Check sheet for the modelled part. Datum: model origin and axes. Units: mm. Round coordinates to 2 decimals unless told otherwise and drop trailing zeros. Loops run counter-clockwise (first coordinate to the right, second up) from the corner with the lowest first, then second, coordinate; pieces in that order, holes last. Notation, with made-up numbers: (79, 42.5) -> (123, 42.5) arc R8 cw to (123, 57.5) -> close; hole circle Ø5 at (-17, 10). An arc over 180 degrees is marked (long way). Use one line per item in the form item = value. Start each with the question number.
(1) Sectioned sample at A-A (y = -50). Record the cut outline in (x, z), and give its area (3 significant figures).
(2) Sectioned sample at D-D (x = 0). State how many separate pieces and enclosed holes the cut face has, and give its area (3 significant figures).
(3) Go/stop test with flat-tipped pins: pin 1 (2.5 mm diameter, centred on x = 0, y = -16.5, fed in from -Z); pin 2 (3 mm diameter, centred on x = -10, z = 4.5, fed in from -Y); pin 3 (3 mm diameter, centred on x = -14, z = 2, fed in from +Y); pin 4 (6 mm diameter, centred on x = 0, y = -50, fed in from -Z). Record where each tip stops, or that it passes through.
(4) Material ranges on probe 1 along Y at (x, z) = (-30, 1.75); probe 2 along Y at (x, z) = (-50, 2.85); probe 3 along X at (y, z) = (20, 4.75), recorded low to high. Write a range as [from, to].
(5) Sectioned sample at C-C (x = -16.5). Record the cut outline in (y, z).
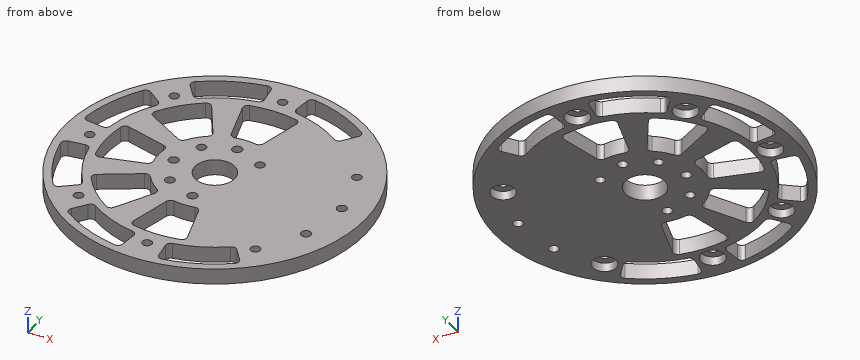
from build123d import *

# Parameters (mm, degrees)
SKETCH1_R                = 60.5
SKETCH1_R_2              = 1.89865
SKETCH1_R_3              = 1.9939
SKETCH1_R_4              = 8
BOSS_EXTRUDE1_DEPTH      = 6.35
CUT_EXTRUDE1_DEPTH       = 86.795235882
FILLET1_R                = 2
CIRPATTERN1_COUNT        = 8
FILLET1_OF_CIRPATTERN1_R = 2
CUT_EXTRUDE2_DEPTH       = 86.795235882
FILLET2_R                = 2
CIRPATTERN3_COUNT        = 8
FILLET2_OF_CIRPATTERN3_R = 2
SKETCH4_R                = 4.7625
SKETCH4_R_2              = 1.89865
CUT_EXTRUDE3_DEPTH       = 3.571875


with BuildPart() as part:
    # Sketch1 → Boss-Extrude1 (new body)
    with BuildSketch(Plane.XY):
        Circle(SKETCH1_R)
        with Locations((45.315389352, 21.130913087)):
            Circle(SKETCH1_R_2, mode=Mode.SUBTRACT)
        with Locations((49.978847504, 1.454235937)):
            Circle(SKETCH1_R_3, mode=Mode.SUBTRACT)
        Circle(SKETCH1_R_4, mode=Mode.SUBTRACT)
        with Locations((46.467376211, -18.460307366)):
            Circle(SKETCH1_R_3, mode=Mode.SUBTRACT)
        with Locations((0, -16.5)):
            Circle(SKETCH1_R_3, mode=Mode.SUBTRACT)
        with Locations((0, -50)):
            Circle(SKETCH1_R_2, mode=Mode.SUBTRACT)
        with Locations((-16.5, 0)):
            Circle(SKETCH1_R_3, mode=Mode.SUBTRACT)
        with Locations((-11.66726189, -11.66726189)):
            Circle(SKETCH1_R_2, mode=Mode.SUBTRACT)
        with Locations((0, 16.5)):
            Circle(SKETCH1_R_3, mode=Mode.SUBTRACT)
        with Locations((-11.66726189, 11.66726189)):
            Circle(SKETCH1_R_2, mode=Mode.SUBTRACT)
        with Locations((11.66726189, 11.66726189)):
            Circle(SKETCH1_R_2, mode=Mode.SUBTRACT)
        with Locations((-35.355339059, -35.355339059)):
            Circle(SKETCH1_R_2, mode=Mode.SUBTRACT)
        with Locations((-50, 0)):
            Circle(SKETCH1_R_2, mode=Mode.SUBTRACT)
        with Locations((-35.355339059, 35.355339059)):
            Circle(SKETCH1_R_2, mode=Mode.SUBTRACT)
        with Locations((0, 50)):
            Circle(SKETCH1_R_2, mode=Mode.SUBTRACT)
        with Locations((35.355339059, -35.355339059)):
            Circle(SKETCH1_R_2, mode=Mode.SUBTRACT)
    extrude(amount=BOSS_EXTRUDE1_DEPTH)

    # Sketch2 → Cut-Extrude1 (cut, through all)
    with BuildSketch(Plane.XY.offset(6.35)):
        with BuildLine():
            Line((-22.071405131, 5.914015181), (-42.162662318, 11.297451319))
            ThreePointArc((-42.162662318, 11.297451319), (-43.65, 0), (-42.162662318, -11.297451319))
            Line((-42.162662318, -11.297451319), (-22.071405131, -5.914015181))
            ThreePointArc((-22.071405131, -5.914015181), (-22.85, 0), (-22.071405131, 5.914015181))
        make_face()
    cut_extrude1 = extrude(amount=-CUT_EXTRUDE1_DEPTH, mode=Mode.SUBTRACT)

    # Fillet1
    fillet1_edges = [part.edges().sort_by_distance(p)[0] for p in [
        (-42.162662318, -11.297451319, 3.175),
        (-42.162662318, 11.297451319, 3.175),
        (-22.071405131, 5.914015181, 3.175),
        (-22.071405131, -5.914015181, 3.175),
    ]]
    fillet(fillet1_edges, radius=FILLET1_R)

    # CirPattern1: Cut-Extrude1 ×8 about axis, 3 skipped
    cirpattern1_axis = Axis((0, 0, 0), (0, 0, -1))
    add([cut_extrude1.rotate(cirpattern1_axis, i * 360 / CIRPATTERN1_COUNT) for i in range(1, CIRPATTERN1_COUNT) if i not in (3, 4, 5)], mode=Mode.SUBTRACT)

    # Fillet1 of CirPattern1
    fillet1_of_cirpattern1_edges = [part.edges().sort_by_distance(p)[0] for p in [
        (-37.802008875, 21.825, 3.175),
        (-21.825, 37.802008875, 3.175),
        (-11.425, 19.788680476, 3.175),
        (-19.788680476, 11.425, 3.175),
        (-11.297451319, 42.162662318, 3.175),
        (11.297451319, 42.162662318, 3.175),
        (5.914015181, 22.071405131, 3.175),
        (-5.914015181, 22.071405131, 3.175),
        (11.297451319, -42.162662318, 3.175),
        (-11.297451319, -42.162662318, 3.175),
        (-5.914015181, -22.071405131, 3.175),
        (5.914015181, -22.071405131, 3.175),
        (-21.825, -37.802008875, 3.175),
        (-37.802008875, -21.825, 3.175),
        (-19.788680476, -11.425, 3.175),
        (-11.425, -19.788680476, 3.175),
    ]]
    fillet(fillet1_of_cirpattern1_edges, radius=FILLET1_OF_CIRPATTERN1_R)

    # Sketch3 → Cut-Extrude2 (cut, through all)
    with BuildSketch(Plane.XY.offset(6.35)):
        with BuildLine():
            Line((-45.478980232, 34.897248918), (-37.148770159, 28.505253913))
            ThreePointArc((-37.148770159, 28.505253913), (-43.26065911, 17.91915172), (-46.424405634, 6.111888951))
            Line((-46.424405634, 6.111888951), (-56.834576678, 7.482413969))
            ThreePointArc((-56.834576678, 7.482413969), (-52.961394201, 21.93732776), (-45.478980232, 34.897248918))
        make_face()
    cut_extrude2 = extrude(amount=-CUT_EXTRUDE2_DEPTH, mode=Mode.SUBTRACT)

    # Fillet2
    fillet2_edges = [part.edges().sort_by_distance(p)[0] for p in [
        (-56.834576678, 7.482413969, 3.175),
        (-45.478980232, 34.897248918, 3.175),
        (-37.148770159, 28.505253913, 3.175),
        (-46.424405634, 6.111888951, 3.175),
    ]]
    fillet(fillet2_edges, radius=FILLET2_R)

    # CirPattern3: Cut-Extrude2 ×8 about axis, 2 skipped
    cirpattern3_axis = Axis((0, 0, 0), (0, 0, -1))
    add([cut_extrude2.rotate(cirpattern3_axis, i * 360 / CIRPATTERN3_COUNT) for i in range(1, CIRPATTERN3_COUNT) if i not in (3, 4)], mode=Mode.SUBTRACT)

    # Fillet2 of CirPattern3
    fillet2_of_cirpattern3_edges = [part.edges().sort_by_distance(p)[0] for p in [
        (-34.897248918, 45.478980232, 3.175),
        (-7.482413969, 56.834576678, 3.175),
        (-6.111888951, 46.424405634, 3.175),
        (-28.505253913, 37.148770159, 3.175),
        (7.482413969, 56.834576678, 3.175),
        (34.897248918, 45.478980232, 3.175),
        (28.505253913, 37.148770159, 3.175),
        (6.111888951, 46.424405634, 3.175),
        (34.897248918, -45.478980232, 3.175),
        (7.482413969, -56.834576678, 3.175),
        (6.111888951, -46.424405634, 3.175),
        (28.505253913, -37.148770159, 3.175),
        (-7.482413969, -56.834576678, 3.175),
        (-34.897248918, -45.478980232, 3.175),
        (-28.505253913, -37.148770159, 3.175),
        (-6.111888951, -46.424405634, 3.175),
        (-45.478980232, -34.897248918, 3.175),
        (-56.834576678, -7.482413969, 3.175),
        (-46.424405634, -6.111888951, 3.175),
        (-37.148770159, -28.505253913, 3.175),
    ]]
    fillet(fillet2_of_cirpattern3_edges, radius=FILLET2_OF_CIRPATTERN3_R)

    # Sketch4 → Cut-Extrude3 (cut)
    # profile 1 of 7: a face of its own
    with BuildSketch(Plane(origin=(0, 0, 0), x_dir=(-1, 0, 0), z_dir=(0, 0, -1))):
        with Locations((0, 50)):
            Circle(SKETCH4_R)
        with Locations((0, 50)):
            Circle(SKETCH4_R_2, mode=Mode.SUBTRACT)
    # profile 2 of 7: a face of its own
    with BuildSketch(Plane(origin=(0, 0, 0), x_dir=(-1, 0, 0), z_dir=(0, 0, -1))):
        with Locations((35.355339059, 35.355339059)):
            Circle(SKETCH4_R)
        with Locations((35.355339059, 35.355339059)):
            Circle(SKETCH4_R_2, mode=Mode.SUBTRACT)
    # profile 3 of 7: a face of its own
    with BuildSketch(Plane(origin=(0, 0, 0), x_dir=(-1, 0, 0), z_dir=(0, 0, -1))):
        with Locations((50, 0)):
            Circle(SKETCH4_R)
        with Locations((50, 0)):
            Circle(SKETCH4_R_2, mode=Mode.SUBTRACT)
    # profile 4 of 7: a face of its own
    with BuildSketch(Plane(origin=(0, 0, 0), x_dir=(-1, 0, 0), z_dir=(0, 0, -1))):
        with Locations((35.355339059, -35.355339059)):
            Circle(SKETCH4_R)
        with Locations((35.355339059, -35.355339059)):
            Circle(SKETCH4_R_2, mode=Mode.SUBTRACT)
    # profile 5 of 7: a face of its own
    with BuildSketch(Plane(origin=(0, 0, 0), x_dir=(-1, 0, 0), z_dir=(0, 0, -1))):
        with Locations((0, -50)):
            Circle(SKETCH4_R)
        with Locations((0, -50)):
            Circle(SKETCH4_R_2, mode=Mode.SUBTRACT)
    # profile 6 of 7: a face of its own
    with BuildSketch(Plane(origin=(0, 0, 0), x_dir=(-1, 0, 0), z_dir=(0, 0, -1))):
        with Locations((-35.355339059, -35.355339059)):
            Circle(SKETCH4_R)
        with Locations((-35.355339059, -35.355339059)):
            Circle(SKETCH4_R_2, mode=Mode.SUBTRACT)
    # profile 7 of 7: a face of its own
    with BuildSketch(Plane(origin=(0, 0, 0), x_dir=(-1, 0, 0), z_dir=(0, 0, -1))):
        with Locations((-45.315389352, 21.130913087)):
            Circle(SKETCH4_R)
        with Locations((-45.315389352, 21.130913087)):
            Circle(SKETCH4_R_2, mode=Mode.SUBTRACT)
    extrude(amount=-CUT_EXTRUDE3_DEPTH, mode=Mode.SUBTRACT)


solid = part.part
Checks:
q1.outline = (-34.06, 0) -> (-28.04, 0) -> (-28.04, 6.35) -> (-34.06, 6.35) -> close; (-6.58, 0) -> (-4.76, 0) -> (-4.76, 3.57) -> (-1.9, 3.57) -> (-1.9, 6.35) -> (-6.58, 6.35) -> close; (1.9, 3.57) -> (4.76, 3.57) -> (4.76, 0) -> (6.58, 0) -> (6.58, 6.35) -> (1.9, 6.35) -> close; (28.04, 0) -> (34.06, 0) -> (34.06, 6.35) -> (28.04, 6.35) -> close
q1.area = 116 mm2
q2.separate_pieces = 8
q2.enclosed_holes = 0
q2.area = 263 mm2
q3.pin_1 = through
q3.pin_2 = -59.9
q3.pin_3 = 59.19
q3.pin_4 = 3.57
q4.probe_1 = [-52.54, -48.85], [-39.1, -31.71], [-17.32, -8.04], [8.04, 17.32], [31.71, 39.1], [48.85, 52.54]
q4.probe_2 = [-34.06, -28.04], [-6.58, -4.76], [4.76, 6.58], [28.04, 34.06]
q4.probe_3 = [-57.1, -53.72], [-42.34, -34.64], [-12.17, 43.79], [46.84, 57.1]
q5.outline = (-58.21, 0) -> (-54.9, 0) -> (-54.9, 6.35) -> (-58.21, 6.35) -> close; (-43.82, 0) -> (-28.58, 0) -> (-28.58, 6.35) -> (-43.82, 6.35) -> close; (-15.81, 0) -> (-1.99, 0) -> (-1.99, 6.35) -> (-15.81, 6.35) -> close; (1.99, 0) -> (15.81, 0) -> (15.81, 6.35) -> (1.99, 6.35) -> close; (28.58, 0) -> (43.82, 0) -> (43.82, 6.35) -> (28.58, 6.35) -> close; (54.9, 0) -> (58.21, 0) -> (58.21, 6.35) -> (54.9, 6.35) -> close
